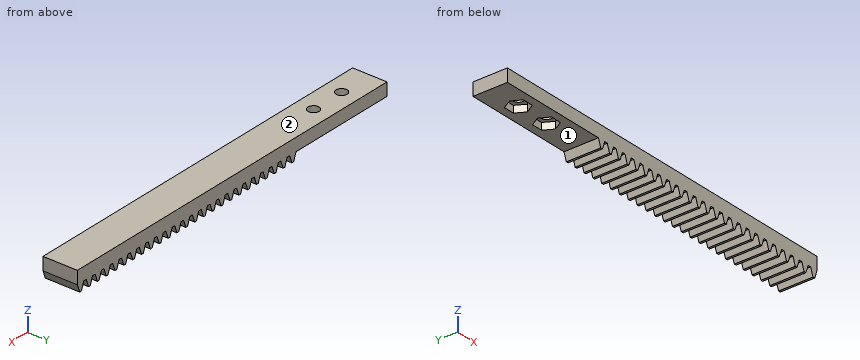
from build123d import *

# Parameters (mm, degrees)
SKETCH_1_W             = 110
SKETCH_1_H             = 3.75
EXTRUDE_1_DEPTH        = 10
EXTRUDE_2_DEPTH        = 10
PATTERN_LINEAR_1_COUNT = 25
PATTERN_LINEAR_1_PITCH = 3.142
SKETCH_2_R             = 1.6
CUT_EXTRUDE_1_DEPTH    = 10
CUT_EXTRUDE_2_DEPTH    = 2


with BuildPart() as part:
    # Sketch 1 → Extrude 1 (new body)
    with BuildSketch(Plane(origin=(0, 0, 0), x_dir=(1, 0, 0), z_dir=(0, 1, 0))):
        with Locations((55, 1.875)):
            Rectangle(SKETCH_1_W, SKETCH_1_H)
    extrude(amount=EXTRUDE_1_DEPTH)

    # Sketch 1_5 → Extrude 2 (add)
    with BuildSketch(Plane(origin=(0, 0, 0), x_dir=(1, 0, 0), z_dir=(0, 1, 0))):
        Polygon((107.747407554, 3.75), (110, 3.75), (109.181203777, 5.999624134), (108.566203777, 5.999624134), align=None)
    extrude_2 = extrude(amount=EXTRUDE_2_DEPTH)

    # Pattern Linear 1: Extrude 2 ×25
    with Locations(*[(-i * PATTERN_LINEAR_1_PITCH, 0, 0) for i in range(1, PATTERN_LINEAR_1_COUNT)]):
        add(extrude_2)

    # Sketch 2 → Cut-Extrude 1 (cut)
    with BuildSketch(Plane(origin=(0, 0, -3.75), x_dir=(-1, 0, 0), z_dir=(0, 0, -1))):
        with Locations((-10, 5)):
            Circle(SKETCH_2_R)
        with Locations((-20, 5)):
            Circle(SKETCH_2_R)
    extrude(amount=-CUT_EXTRUDE_1_DEPTH, mode=Mode.SUBTRACT)

    # Sketch 3 → Cut-Extrude 2 (cut)
    with BuildSketch(Plane(origin=(0, 0, -3.75), x_dir=(-1, 0, 0), z_dir=(0, 0, -1))):
        Polygon((-21.58771324, 7.75), (-23.175426481, 5), (-21.58771324, 2.25), (-18.41228676, 2.25), (-16.824573519, 5), (-18.41228676, 7.75), align=None)
        Polygon((-11.58771324, 7.75), (-13.175426481, 5), (-11.58771324, 2.25), (-8.41228676, 2.25), (-6.824573519, 5), (-8.41228676, 7.75), align=None)
    extrude(amount=-CUT_EXTRUDE_2_DEPTH, mode=Mode.SUBTRACT)


solid = part.part
Geometry: final body of the model. Coordinates: model frame, mm. Face numbers are marked on the shaded views. A direction names the side the tool comes from. Give positions to 0.01 mm unless a question says otherwise; leave off trailing zeros. Loops run counter-clockwise (first coordinate to the right, second up) from the corner with the lowest first, then second, coordinate; pieces in that order, holes last. Notation, with made-up numbers: (12, 6) - (36, 6) arc R26 cw to (36, 34) - close; hole circle Ø1 at (-24, 33.5). An arc over 180 degrees is marked (long way). One line per question, with ' | ' between items. Start each with the question number.
(1) Contact query for a flat-ended pin moving along its axis: pin 1 (2 mm diameter, centred on x = 29.5, y = 7, fed in from -Z). Output: stop coordinate, or through.
(2) Ray query, line 1 (Y direction, x = 10, z = -0.85); line 2 (X direction, y = 6, z = -3.7); line 3 (Z direction, x = 6, y = 9). Return the intervals inside material, ascending. Write a range as from..to.
(3) Reachability of the marked faces 1 and 2 from +Z, -Z, +X, -X, +Y, -Y: full face, straight path, thin tool, end or side. Return the list, or none.
(4) Section query A-A on x = 20. Return loops of the section in (y, z).
The answers:
1) pin 1: z = -3.75
2) line 1: 0..3.4, 6.6..10 | line 2: 0..7.4, 12.6..17.4, 22.6..110 | line 3: -3.75..0
3) face 1: -Z, -X, +Y, -Y | face 2: +Z, +X, -X, +Y, -Y
4) outline: (0, -3.75) - (2.25, -3.75) - (2.25, -1.75) - (3.4, -1.75) - (3.4, 0) - (0, 0) - close; (6.6, -1.75) - (7.75, -1.75) - (7.75, -3.75) - (10, -3.75) - (10, 0) - (6.6, 0) - close
